Read the model definition and answer for the solid it produces. Units are mm, in the model's axes. Face numbers are marked on the shaded views. A direction names the side the tool comes from. Give positions to 0.01 mm unless a question says otherwise; leave off trailing zeros. Order: outer loops, then holes, each group sorted by start corner. A loop starts at its lowest first (then second) coordinate and runs counter-clockwise, first axis right, second up. Notation, with made-up numbers: M 63.5,25 L 119.5,25 A19 cw 119.5,33 Z; hole C 28,-34 d6. An arc over 180 degrees is marked long. One line per item, written item: value.
Autodesk Inventor part; units mm, degrees
ref_plane "工作平面1" through (0, 0, 20) normal (0, 0, 1) x (1, 0, 0)
ref_plane "YZ Plane" through (0, 0, 0) normal (1, 0, 0) x (0, 1, 0)
ref_plane "XZ Plane" through (0, 0, 0) normal (0, 1, 0) x (-1, 0, 0)
sketch "草图1" plane through (0, 0, 0) normal (0, 0, 1) x (1, 0, 0)
  line L0 (-10, 0) -> (10, 0)
  line L1 (10, 0) -> (10, 24)
  line L2 (10, 24) -> (8, 24)
  line L3 (8, 24) -> (5.6906, 20)
  line L4 (5.6906, 20) -> (-5.6906, 20)
  line L5 (-5.6906, 20) -> (-8, 24)
  line L6 (-8, 24) -> (-10, 24)
  line L7 (-10, 24) -> (-10, 0)
  line L8 (-14, 0) -> (14, 0)
  point P0 (0, 0)
  point P1 (0, 0)
  dimension "d1" = 24
  dimension "d2" = 4
  dimension "d4" = 20
  dimension "d5" = 2
  dimension "d6" = 120
  dimension "d7" = 120
  dimension "d8" = 2
revolve "旋转1" add sketch "草图1" angle 360 about axis through (-10, 0, 0) along (1, 0, 0)
sketch "草图2" plane through (10, 0, 0) normal (1, 0, 0) x (0, 0, -1)
  circle A0 centre (0, 0) radius 7.5
  dimension "d10" = 15
extrude "拉伸1" cut sketch "草图2" against normal through all
ref_plane "工作平面1" through (0, 0, 20) normal (0, 0, 1) x (1, 0, 0)
sketch "草图3" plane through (0, 0, 20) normal (0, 0, 1) x (1, 0, 0)
  circle A0 centre (0, 0) radius 2
  dimension "d13" = 4
extrude "拉伸2" cut sketch "草图3" against normal up to surface
thread "螺纹1"
properties part number "砂轮电机皮带轮"
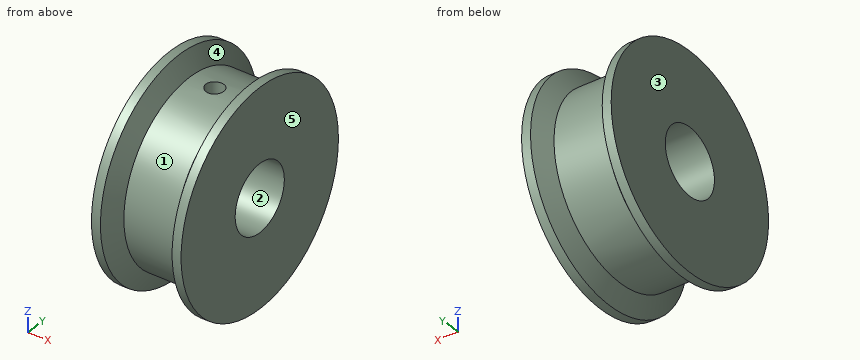
1) Find section B-B, the plane y = 0. Write down the section's boundary in (x, z), plus the area to 3 significant figures.
Reported:
outline: M -10,-24 L -8,-24 L -5.69,-20 L 5.69,-20 L 8,-24 L 10,-24 L 10,-7.5 L -10,-7.5 Z; M -10,7.5 L -2,7.5 L -2,20 L -5.69,20 L -8,24 L -10,24 Z; M 2,7.5 L 10,7.5 L 10,24 L 8,24 L 5.69,20 L 2,20 Z
area: 500 mm^2
2) Consider probe 1 along Z at (x, y) = (3, 0); probe 2 along X at (y, z) = (0, 14); probe 3 along Z at (x, y) = (-0.5, -3). Determine where each line is inside the solid, lowest interval first.
Reported:
probe 1: z = -20 to -7.5, 7.5 to 20
probe 2: x = -10 to -2, 2 to 10
probe 3: z = -19.77 to -6.87, 6.87 to 19.77
3) Determine the mould class of the marked faces 3, 4 and 5 for opening direction X: +X half, -X half, draft (parallel to the pull), parting line (faces both ways), or undercut.
Reported:
face 3: -X half
face 4: undercut
face 5: +X half
4) Which of the six approach directions +Z, -Z, +X, -X, +Y, -Y give full straight-line access (tool end or side, diameter ignored) to the marked faces 1 and 2?
Reported:
face 1: none
face 2: +X, -X
5) Find section A-A, the plane z = 0. Write down the section's boundary in (x, y).
Reported:
outline: M -10,-24 L -8,-24 L -5.69,-20 L 5.69,-20 L 8,-24 L 10,-24 L 10,-7.5 L -10,-7.5 Z; M -10,7.5 L 10,7.5 L 10,24 L 8,24 L 5.69,20 L -5.69,20 L -8,24 L -10,24 Z
6) Find section D-D, the plane x = 0. Write down the section's boundary in (y, z), plus the area to 3 significant figures.
Reported:
outline: M -2,7.23 L -2,19.9 A20 ccw long 2,19.9 L 2,7.23 A7.5 cw long Z
area: 1,030 mm^2
7) Each of these flat-tipped pins is pushed along its axis until it touches: pin 1 Ø1.5 at (x, y) = (7.5, 1.5) entering from +Z; pin 2 Ø5 at (x, y) = (8, -6.5) entering from -Z; pin 3 Ø1 at (x, z) = (0, 9) entering from +Y. Where does it stop, or does it pass through?
Reported:
pin 1: stops at z = 23.98
pin 2: stops at z = -23.66
pin 3: stops at y = 18.1
8) Find section C-C, the plane x = -4.75. Write down the section's boundary in (y, z).
Reported:
outline: C 0,0 d40; hole C 0,0 d15
